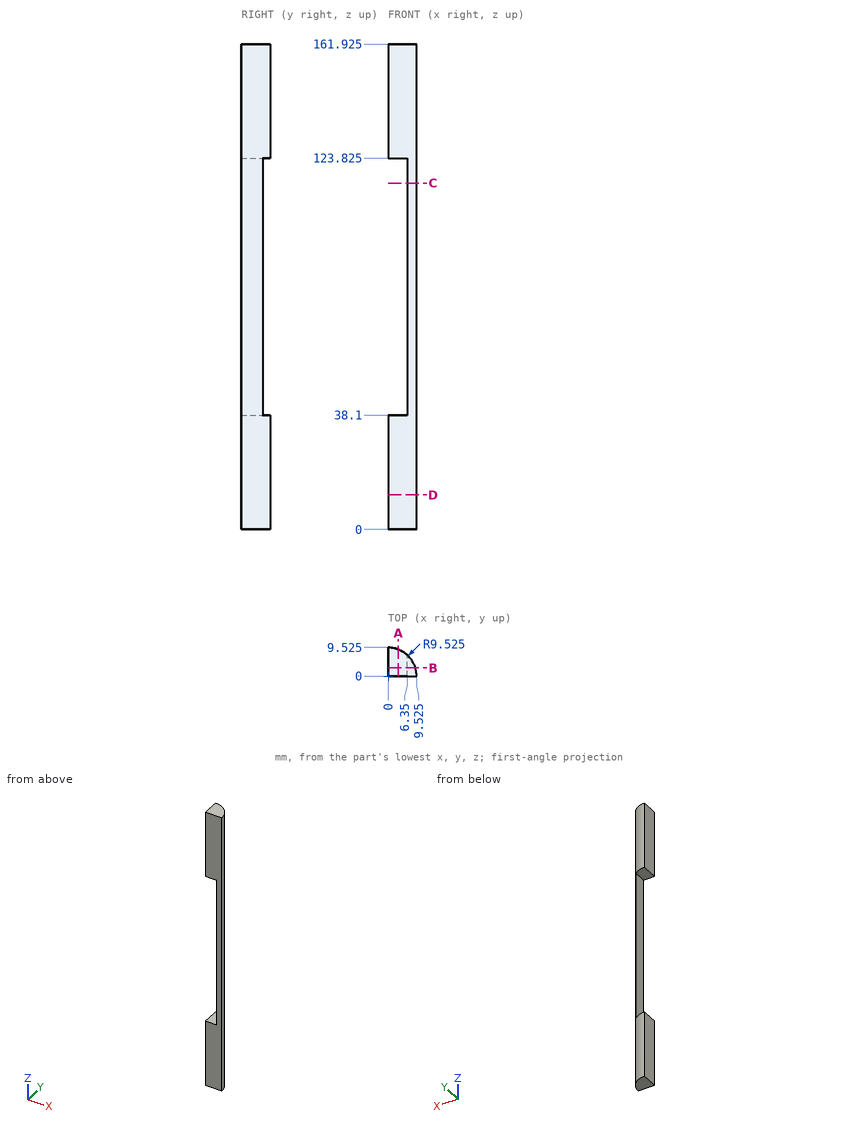
Answer from the drawing. Dimensions are ordinates in mm from the lowest x, y and z of the part. Give positions to 0.01 mm unless a question says otherwise; leave off trailing zeros. Order: outer loops, then holes, each group sorted by start corner. A loop starts at its lowest first (then second) coordinate and runs counter-clockwise, first axis right, second up. Notation, with made-up numbers: (28, 45.5) - (71, 45.5) arc R28 ccw to (71, 74.5) - close; hole circle Ø5 at (78.5, -16). An arc over 180 degrees is marked (long way). Use one line per item in the form item = value.
1) Find section C-C on z = 115.5. Determine the outline of the cut face in (x, y) (3 decimals), and give its area (3 significant figures).
Verdict:
outline = (6.35, 0) - (9.525, 0) arc R9.525 ccw to (6.35, 7.1) - close
area = 15.6 mm^2
2) Consider probe 1 along Z at (x, y) = (2.25, 6.75) (3 decimals); probe 2 along X at (y, z) = (8.25, 11); probe 3 along X at (y, z) = (1.25, 87.5). Determine where each line is inside the solid, lowest interval first. Write a range as [from, to].
Verdict:
probe_1 = [0, 38.1], [123.825, 161.925]
probe_2 = [0, 4.76]
probe_3 = [6.35, 9.44]
3) Find section B-B on y = 2.75. Determine the outline of the cut face in (x, z) (3 decimals).
Verdict:
outline = (0, 0) - (9.119, 0) - (9.119, 161.925) - (0, 161.925) - (0, 123.825) - (6.35, 123.825) - (6.35, 38.1) - (0, 38.1) - close
4) Find section A-A on x = 3.5. Determine the outline of the cut face in (y, z) (3 decimals).
Verdict:
outline = (0, 0) - (8.859, 0) - (8.859, 38.1) - (0, 38.1) - close; (0, 123.825) - (8.859, 123.825) - (8.859, 161.925) - (0, 161.925) - close
5) Each of these flat-tipped pins is pushed along its axis until it touches: pin 1 (3.5 mm diameter, centred on y = 5, z = 69.5, fed in from -X); pin 2 (1.5 mm diameter, centred on x = 8, y = 4.5, fed in from -Z); pin 3 (1.5 mm diameter, centred on x = 8, y = 6.5, fed in from +Z). Where does it stop, or does it pass through?
Verdict:
pin_1 = 6.35
pin_2 = 0
pin_3 = through
6) Find section D-D on z = 11.5. Determine the outline of the cut face in (x, y) (3 decimals), and give its area (3 significant figures).
Verdict:
outline = (0, 0) - (9.525, 0) arc R9.525 ccw to (0, 9.525) - close
area = 71.3 mm^2
